For this review, take the finished solid that the model builds, in its own axes (mm). Face numbers are marked on the shaded views. A direction names the side the tool comes from. Coordinates: 2 decimals unless noted, no trailing zeros. Order: outer loops, then holes, each group sorted by start corner. A loop starts at its lowest first (then second) coordinate and runs counter-clockwise, first axis right, second up. Notation, with made-up numbers: (-10, 54.25) -> (12, 54.25) arc R20 cw to (12, 87.25) -> close; hole circle Ø5 at (13.25, -13). An arc over 180 degrees is marked (long way). Write item = value, one per line. Start each with the question number.
1) Consider section C-C on z = 64.5. Give the boundary of the cut face in (x, y).
2) Wall thickness on probe 1 along Z at (x, y) = (0, 0); probe 2 along Z at (x, y) = (1, 0); probe 3 along X at (y, z) = (-1.5, 5): over which ranges is each line inside the solid? List them lowest first. Write a range as [from, to].
3) Consider section B-B on x = 0. Give the boundary of the cut face in (y, z), and give its area (3 significant figures).
4) Consider section D-D on z = -134. Give the boundary of the cut face in (x, y).
5) Machinability: for the marked faces 1 and 2, which of the approach directions +Z, -Z, +X, -X, +Y, -Y give a long, thin tool a straight path to every point of the face, cutting with its end or side? Answer none if there is none.
6) Consider section A-A on y = 0. Give the boundary of the cut face in (x, z).
7) Insertion check: pin 1 Ø8 at (x, z) = (-9.5, 102.5) entering from +Y; pin 2 Ø2 at (y, z) = (-11, 5.5) entering from -X; pin 3 Ø4 at (x, z) = (7, 14.5) entering from +Y; pin 4 Ø8 at (y, z) = (0, 128.12) entering from -X. Each pin has a flat end and moves straight along its axis. Give the tip position at first contact, or say it passes through.
Autodesk Inventor part; units mm, degrees
ref_plane "YZ Plane" through (0, 0, 0) normal (1, 0, 0) x (0, 1, 0)
ref_plane "XZ Plane" through (0, 0, 0) normal (0, 1, 0) x (-1, 0, 0)
ref_plane "XY Plane" through (0, 0, 0) normal (0, 0, 1) x (1, 0, 0)
sketch "Sketch1" plane through (0, 0, 0) normal (0, 0, 1) x (1, 0, 0)
  circle A0 centre (0, 0) radius 17.5
  dimension "D" = 35
extrude "Extrusion1" add sketch "Sketch1" along normal blind 121.5
sketch "Sketch2" plane through (0, 0, 0) normal (0, 1, 0) x (-1, 0, 0)
  line L0 (17.5, 121.5) -> (-17.5, 121.5)
  line L1 (0, 121.5) -> (0, 139)
  arc A0 (0, 139) -> (-17.5, 121.5) centre (0, 121.5) ccw
  line L2 (-17.5, 0) -> (-17.5, 121.5) construction
  point P0 (0, 0)
  dimension "d3" = 17.5
revolve "Revolution1" add sketch "Sketch2" angle 360 about axis through (0, 0, 121.5) along (0, 0, 1)
sketch "Sketch3" plane through (0, 0, 0) normal (0, 0, -1) x (-1, 0, 0)
  circle A0 centre (0, 0) radius 17.5
  circle A1 centre (0, 0) radius 14
  dimension "d5" = 28
extrude "Extrusion2" add sketch "Sketch3" along normal blind 178 contours A1
sketch "Sketch4" plane through (0, 0, -178) normal (0, 0, -1) x (-1, 0, 0)
  circle A0 centre (0, 0) radius 10
  dimension "d8" = 20
extrude "Extrusion3" add sketch "Sketch4" along normal blind 20
fillet "Fillet1" radius 10 1 edges at (10, 0, -198)
sketch "Sketch5" plane through (0, 0, 0) normal (1, 0, 0) x (0, 1, 0)
  circle A0 centre (0, 128.1186) radius 5
  line L0 (-10, -188) -> (10, -188)
  circle A1 centre (0, -188) radius 5
  point P0 (0, 0)
  dimension "d12" = 10
  dimension "d13" = 10
extrude "Extrusion4" cut sketch "Sketch5" along normal through all both and the other way through all
properties part number "ANT-35"
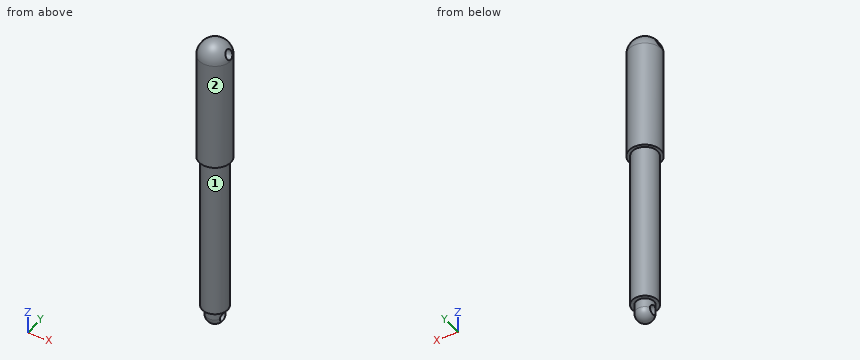
Answer sheet:
q1.outline = circle Ø35 at (0, 0)
q2.probe_1 = [-198, -193], [-183, 123.12], [133.12, 139]
q2.probe_2 = [-197.95, -193], [-183, 123.12], [133.12, 138.97]
q2.probe_3 = [-17.44, 17.44]
q3.outline = (-17.5, 0) -> (-14, 0) -> (-14, -178) -> (-10, -178) -> (-10, -188) arc R10 ccw to (10, -188) -> (10, -178) -> (14, -178) -> (14, 0) -> (17.5, 0) -> (17.5, 121.5) arc R17.5 ccw to (-17.5, 121.5) -> close; hole circle Ø10 at (0, -188); hole circle Ø10 at (0, 128.12)
q3.area = 9,920 mm2
q4.outline = circle Ø28 at (0, 0)
q5.face_1 = -Z
q5.face_2 = +Z, -Z
q6.outline = (-17.5, 0) -> (-14, 0) -> (-14, -178) -> (-10, -178) -> (-10, -183) -> (10, -183) -> (10, -178) -> (14, -178) -> (14, 0) -> (17.5, 0) -> (17.5, 121.5) arc R17.5 ccw to (17.42, 123.12) -> (-17.42, 123.12) arc R17.5 ccw to (-17.5, 121.5) -> close; (-13.09, 133.12) -> (13.09, 133.12) arc R17.5 ccw to start; (-8.66, -193) arc R10 ccw to (8.66, -193) -> close
q7.pin_1 = 16.61
q7.pin_2 = -14.36
q7.pin_3 = 16.77
q7.pin_4 = through
